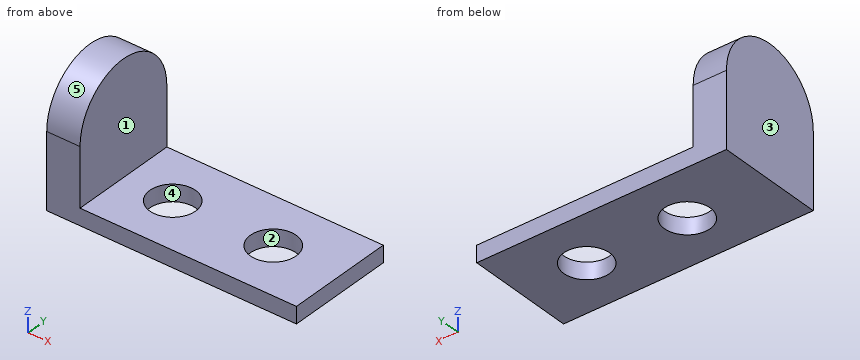
from build123d import *

# Parameters (mm, degrees)
F1_DEPTH = 82.55
F3_DEPTH = 25.4
F4_R     = 17.4625
F5_DEPTH = 12.7


with BuildPart() as f1:
    # F0 (on Front) → F1 (new body)
    with BuildSketch(Plane.XZ):
        Polygon((0, 127), (0, 0), (190.5, 0), (190.5, 12.7), (25.4, 12.7), (25.4, 127), align=None)
    extrude(amount=F1_DEPTH)

    # F2 (on face) → F3 (cut)
    with BuildSketch(Plane(origin=(0, 0, 0), x_dir=(0, -1, 0), z_dir=(-1, 0, 0))):
        with BuildLine():
            Line((0, 127), (0, 57.15))
            ThreePointArc((0, 57.15), (41.275, 98.425), (82.55, 57.15))
            Line((82.55, 57.15), (82.55, 127))
            Line((82.55, 127), (0, 127))
        make_face()
    extrude(amount=-F3_DEPTH, mode=Mode.SUBTRACT)

    # F4 (on face) → F5 (cut)
    with BuildSketch(Plane.XY.offset(12.7)):
        with Locations((63.5, -41.918826)):
            Circle(F4_R)
        with Locations((139.7, -41.275)):
            Circle(F4_R)
    extrude(amount=-F5_DEPTH, mode=Mode.SUBTRACT)


solid = f1.part
Geometry check sheet. Reference: the model listing, model coordinates, mm. Face numbers are marked on the shaded views. A direction names the side the tool comes from. Round coordinates to 2 decimals unless told otherwise and drop trailing zeros. Order: outer loops, then holes, each group sorted by start corner. A loop starts at its lowest first (then second) coordinate and runs counter-clockwise, first axis right, second up. Notation, with made-up numbers: M 75,57 L 89,57 A6 ccw 89,64 Z; hole C 30,-26 d3. An arc over 180 degrees is marked long. Write each question's results on one line, items separated by ' | '. Start each with the question number.
1. Draft check along X on the marked faces 3, 4 and 5. Enter one of: pulls with the +X half, pulls with the -X half, needs draft (parallel to the pull), parting line crosses it, or undercut.
2. Cross-section at D-D on z = 63.5. Record the boundary of the cut face in (x, y), plus the area to 3 significant figures.
3. Cross-section at A-A on x = 139.7. Record the boundary of the cut face in (y, z), plus the area to 3 significant figures.
4. Set-up check for the marked faces 1 and 2: record each of +Z, -Z, +X, -X, +Y, -Y from which the full face is reachable in a straight line by a thin tool's end or side.
5. Material ranges on L1, parallel to Y at x = 139.7, z = 3.5; L2, parallel to Z at x = 36, y = -17; L3, parallel to X at y = -48, z = 28, recorded low to high. Write a range as from..to.
6. Go/stop test with flat-tipped pins: P1, Ø6, axis at y = -40, z = 38.5, coming from the +X side; P2, Ø1.5, axis at x = 59.5, y = -73.5, coming from the +Z side. Record where each tip stops, or that it passes through.
7. Cross-section at C-C on y = -6. Record the boundary of the cut face in (x, z), plus the area to 3 significant figures.
8. Cross-section at B-B on y = -53. Record the boundary of the cut face in (x, z), plus the area to 3 significant figures.
Resolved:
1) face 3: pulls with the -X half | face 4: undercut | face 5: needs draft
2) outline: M 0,-82.06 L 25.4,-82.06 L 25.4,-0.49 L 0,-0.49 Z | area: 2,070 mm2
3) outline: M -82.55,0 L -58.74,0 L -58.74,12.7 L -82.55,12.7 Z; M -23.81,0 L 0,0 L 0,12.7 L -23.81,12.7 Z | area: 605 mm2
4) face 1: +Z, +X, +Y, -Y | face 2: +Z, -Z
5) L1: -82.55..-58.74, -23.81..0 | L2: 0..12.7 | L3: 0..25.4
6) P1: x = 25.4 | P2: z = 12.7
7) outline: M 0,0 L 190.5,0 L 190.5,12.7 L 25.4,12.7 L 25.4,78.58 L 0,78.58 Z | area: 4,090 mm2
8) outline: M 0,0 L 50,0 L 50,12.7 L 25.4,12.7 L 25.4,96.72 L 0,96.72 Z; M 77,0 L 126.76,0 L 126.76,12.7 L 77,12.7 Z; M 152.64,0 L 190.5,0 L 190.5,12.7 L 152.64,12.7 Z | area: 3,880 mm2
